Autodesk Fusion 360 part; units mm, degrees
sketch "Sketch1" plane through (0, 0, 0) normal (0, 0, 1) x (1, 0, 0)
  line L0 (0, 0) -> (40, 0)
  line L1 (40, 0) -> (40, 17)
  line L2 (40, 17) -> (0, 17)
  line L3 (0, 17) -> (0, 0)
  dimension "d1" = 40
  dimension "d2" = 17
extrude "Extrude1" add sketch "Sketch1" along normal blind 5
sketch "Sketch2" plane through (0, 0, 5) normal (0, 0, 1) x (-1, 0, 0)
  line L0 (0, -17) -> (0, 0)
  line L1 (0, 0) -> (-40, 0)
  line L2 (-40, 0) -> (-40, -17)
  line L3 (-40, -17) -> (0, -17)
  line L4 (0, 0) -> (-40, 0)
  line L5 (-40, 0) -> (-40, -7)
  line L6 (-40, -7) -> (0, -7)
  line L7 (0, -7) -> (0, 0)
  dimension "d5" = 40
  dimension "d6" = 7
extrude "Extrude2" add sketch "Sketch2" along normal blind 55 contours L0 L1 L2 L4 L5 L6 L7
sketch "Sketch3" plane through (0, 0, 0) normal (0, -1, 0) x (1, 0, 0)
  line L0 (0, 0) -> (40, 0)
  line L1 (40, 0) -> (40, 60)
  line L2 (40, 60) -> (0, 60)
  line L3 (0, 60) -> (0, 0)
  circle A0 centre (20, 40) radius 16
  dimension "d9" = 32
extrude "Extrude3" cut sketch "Sketch3" against normal blind 7 contours A0
sketch "Sketch4" plane through (0, 0, 5) normal (0, 0, 1) x (-1, 0, 0)
  line L0 (0, -7) -> (-40, -7)
  line L1 (-40, -7) -> (-40, -17)
  line L2 (-40, -17) -> (0, -17)
  line L3 (-40, -17) -> (-30, -17)
  line L4 (-30, -17) -> (-30, -7)
  line L5 (-30, -7) -> (-40, -7)
  line L6 (-40, -7) -> (-40, -17)
  circle A0 centre (-30, -12) radius 4.5
  line L7 (-30, -12) -> (-10, -12)
  line L8 (-10, -12) -> (-10, -17)
  line L9 (-10, -17) -> (-30, -17)
  line L10 (-30, -17) -> (-30, -12)
  circle A1 centre (-10, -12) radius 4.5
  line L11 (0, -17) -> (0, -7)
  dimension "d24" = 10
  dimension "d25" = 10
  dimension "d26" = 9
  dimension "d27" = 20
  dimension "d28" = 5
  dimension "d29" = 9
extrude "Extrude7" cut sketch "Sketch4" against normal blind 3 contours L4 A0 L7 | L4 A0 L10 | L4 A0 L7 L10 | L7 L8 A1 | L7 L8 A1
sketch "Sketch7" plane through (0, 0, 5) normal (0, 0, 1) x (-1, 0, 0)
  circle A0 centre (-30, -12) radius 3
  circle A1 centre (-10, -12) radius 3
  dimension "d32" = 6
  dimension "d33" = 6
extrude "Extrude8" cut sketch "Sketch7" against normal blind 5
fillet "Fillet2" radius 3.5 11 edges at (0, 17, 2.5) (40, 7, 32.5) (40, 17, 2.5) (0, 0, 30) (0, 7, 32.5) (0, 3.5, 60) (20, 7, 60) (20, 0, 60) (40, 3.5, 60) (40, 0, 30) (20, 17, 5)
Read the model definition and answer for the solid it produces. Units are mm, in the model's axes. A direction names the side the tool comes from. Round coordinates to 2 decimals unless told otherwise and drop trailing zeros. Write each loop counter-clockwise with the first axis right and the second up, starting at its lowest first coordinate (ties: lowest second). Pieces come first, ordered by that corner, then holes. Notation, with made-up numbers: M 59,-15.5 L 114,-15.5 A13 ccw 114,-8.5 Z; hole C 84,36.25 d10. An arc over 180 degrees is marked long. Use a Markdown table: item, result.
1) For a pull along Y with two mould halves and no side action, classify faces 5 (the cylindrical face through (39.389, 15.476, 1.979)), 6 (the flat face through (7, 13, 2)), 7 (the cylindrical face through (17.917, 3.451, 55.864)) as pulls with the +Y half, pulls with the -Y half, needs draft (parallel to the pull), parting line crosses it, or undercut.
Answers follow:
| item | result |
|---|---|
| face 5 | pulls with the +Y half |
| face 6 | undercut |
| face 7 | needs draft |
2) The part is cut by section B-B (y = 12). Write down the section's boundary in (x, z), plus the area to 3 significant figures.
Answers follow:
| item | result |
|---|---|
| outline | M 0,0 L 7,0 L 7,2 L 5.5,2 L 5.5,5 L 0,5 Z; M 13,0 L 27,0 L 27,2 L 25.5,2 L 25.5,5 L 14.5,5 L 14.5,2 L 13,2 Z; M 33,0 L 40,0 L 40,5 L 34.5,5 L 34.5,2 L 33,2 Z |
| area | 122 mm2 |
3) Flat-ended cylindrical pins translate along their axes: pin 1 (6 mm diameter, centred on x = 30, z = 34.5, fed in from -Y); pin 2 (2.5 mm diameter, centred on x = 9, y = 10.5, fed in from +Z); pin 3 (1 mm diameter, centred on x = 35, z = 15.5, fed in from +Y). Find the tip coordinate at first contact, or state that the pin passes through.
Answers follow:
| item | result |
|---|---|
| pin 1 | passes through |
| pin 2 | stops at z = 2 |
| pin 3 | stops at y = 7 |
4) Straight lines are drawn through the part: line 1 along X through (y, z) = (12, 0.5); line 2 along X through (y, z) = (12, 2.75); line 3 along Y through (x, z) = (10, 3). For each, find the intervals that lie inside material, in ascending order. Write a range as [from, to].
Answers follow:
| item | result |
|---|---|
| line 1 | x = [0, 7], [13, 27], [33, 40] |
| line 2 | x = [0, 5.5], [14.5, 25.5], [34.5, 40] |
| line 3 | y = [0, 7.5], [16.5, 17] |
5) A tool of negligible diameter and unlimited length cuts with its end or side. For faces 1 (the cylindrical face through (36.441, 15.476, 4.389)), 2 (the cylindrical face through (3.478, 15.476, 4.389)), 3 (the flat face through (20, 7, 19)), 4 (the cylindrical face through (5.708, 10.648, 3.521)), from which of +Z, -Z, +X, -X, +Y, -Y can it reach the whole face along a straight path? Write none if from no direction.
Answers follow:
| item | result |
|---|---|
| face 1 | +Z, +X, +Y |
| face 2 | +Z, -X, +Y |
| face 3 | +Z, +X, -X, +Y |
| face 4 | +Z |
